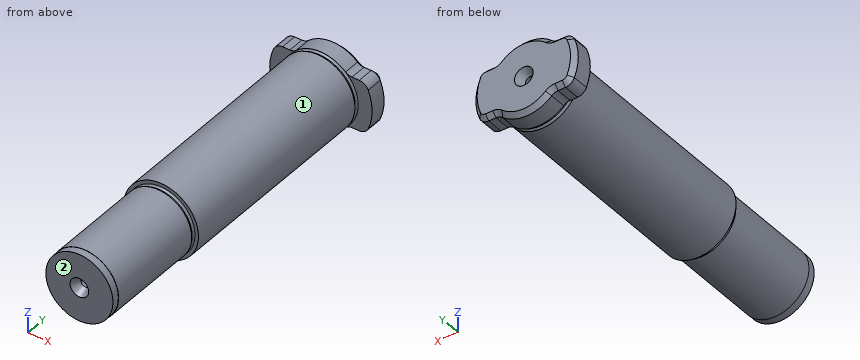
```python
from build123d import *

# Parameters (mm, degrees)
F0_R            = 11.4427
F1_DEPTH        = 2.54
F2_R            = 11.52271
F3_DEPTH        = 35.7378
F4_R            = 12.7
F4_R_2          = 11.52271
F5_DEPTH        = 74.7268
F7_DEPTH        = 7.1374
F8_T1_DEPTH     = 7.1374
F8_T3_DEPTH     = 18.5145836873
F9_SIZE         = 1.524
F13_D           = 3.048
F13_DEPTH       = 12.7
F13_CSINK_D     = 6.35
F13_CSINK_ANGLE = 60
F13_TIP         = 0.9157115834
F15_D           = 3.048
F15_DEPTH       = 12.7
F15_CSINK_D     = 6.35
F15_CSINK_ANGLE = 60
F15_TIP         = 0.9157115834


# Not quite as in the source:
# - a fillet or chamfer that OpenCascade refuses, or shapes differently, is made with other operations: its cross-section is extruded or revolved along the edge and cut away or added


with BuildPart() as f1:
    # F0 (on Front) → F1 (new body)
    with BuildSketch(Plane.XZ):
        Circle(F0_R)
    extrude(amount=-F1_DEPTH)

    # F2 (on face) → F3 (join)
    with BuildSketch(Plane(origin=(0, 2.54, 0), x_dir=(-1, 0, 0), z_dir=(0, 1, 0))):
        Circle(F2_R)
    extrude(amount=F3_DEPTH)

    # F4 (on face) → F5 (join)
    with BuildSketch(Plane(origin=(0, 38.2778, 0), x_dir=(-1, 0, 0), z_dir=(0, 1, 0))):
        Circle(F4_R)
        Circle(F4_R_2, mode=Mode.SUBTRACT)
        Circle(F4_R_2)
    extrude(amount=F5_DEPTH)

    # F6 (on face) → F7 (join)
    with BuildSketch(Plane(origin=(0, 113.0046, 0), x_dir=(-1, 0, 0), z_dir=(0, 1, 0))):
        with BuildLine():
            ThreePointArc((12.7, 0), (11.8067080769, 4.678850755), (9.2524969468, 8.6995))
            ThreePointArc((9.2524969468, 8.6995), (0, 12.7), (-9.2524969468, 8.6995))
            ThreePointArc((-9.2524969468, 8.6995), (-12.7, 0), (-9.2524969468, -8.6995))
            ThreePointArc((-9.2524969468, -8.6995), (0, -12.7), (9.2524969468, -8.6995))
            ThreePointArc((9.2524969468, -8.6995), (11.8067080769, -4.678850755), (12.7, 0))
        make_face()
        with BuildLine():
            ThreePointArc((15.126606354, -8.6995), (17.4498, 0), (15.126606354, 8.6995))
            Line((15.126606354, 8.6995), (9.2524969468, 8.6995))
            ThreePointArc((9.2524969468, 8.6995), (11.8067080769, 4.678850755), (12.7, 0))
            ThreePointArc((12.7, 0), (11.8067080769, -4.678850755), (9.2524969468, -8.6995))
            Line((9.2524969468, -8.6995), (15.126606354, -8.6995))
        make_face()
        with BuildLine():
            ThreePointArc((-9.2524969468, -8.6995), (-12.7, 0), (-9.2524969468, 8.6995))
            Line((-9.2524969468, 8.6995), (-15.126606354, 8.6995))
            ThreePointArc((-15.126606354, 8.6995), (-17.4498, 0), (-15.126606354, -8.6995))
            Line((-15.126606354, -8.6995), (-9.2524969468, -8.6995))
        make_face()
    extrude(amount=F7_DEPTH)

    # F8: fillet of radius 3.302 on 8 edges, made by hand

    # F8_s2 → F8_t1 (join)
    with BuildSketch(Plane.XZ.offset(-120.142)):
        with BuildLine():
            ThreePointArc((-8.4002604126, -9.525), (-9.4168948242, -8.9127618272), (-10.5843281199, -8.6995))
            Line((-10.5843281199, -8.6995), (-9.2524969468, -8.6995))
            ThreePointArc((-9.2524969468, -8.6995), (-8.8360241715, -9.1222078928), (-8.4002604126, -9.525))
        make_face()
        with BuildLine():
            ThreePointArc((8.4002604126, -9.525), (9.4168948242, -8.9127618272), (10.5843281199, -8.6995))
            Line((10.5843281199, -8.6995), (9.2524969468, -8.6995))
            ThreePointArc((9.2524969468, -8.6995), (8.8360241715, -9.1222078928), (8.4002604126, -9.525))
        make_face()
        with BuildLine():
            ThreePointArc((-8.4002604126, 9.525), (-9.4168948242, 8.9127618272), (-10.5843281199, 8.6995))
            Line((-10.5843281199, 8.6995), (-9.2524969468, 8.6995))
            ThreePointArc((-9.2524969468, 8.6995), (-8.8360241715, 9.1222078928), (-8.4002604126, 9.525))
        make_face()
        with BuildLine():
            ThreePointArc((8.4002604126, 9.525), (9.4168948242, 8.9127618272), (10.5843281199, 8.6995))
            Line((10.5843281199, 8.6995), (9.2524969468, 8.6995))
            ThreePointArc((9.2524969468, 8.6995), (8.8360241715, 9.1222078928), (8.4002604126, 9.525))
        make_face()
    extrude(amount=F8_T1_DEPTH)

    # F8_s4 → F8_t3 (cut)
    with BuildSketch(Plane.XZ.offset(-125.8305918437)):
        with BuildLine():
            ThreePointArc((-13.0777382827, -8.6995), (-14.913976773, -8.1418454969), (-16.1299931781, -6.6572396768))
            ThreePointArc((-16.1299931781, -6.6572396768), (-15.6616238106, -7.6947423385), (-15.126606354, -8.6995))
            Line((-15.126606354, -8.6995), (-13.0777382827, -8.6995))
        make_face()
        with BuildLine():
            ThreePointArc((13.0777382827, -8.6995), (14.913976773, -8.1418454969), (16.1299931781, -6.6572396768))
            ThreePointArc((16.1299931781, -6.6572396768), (15.6616238106, -7.6947423385), (15.126606354, -8.6995))
            Line((15.126606354, -8.6995), (13.0777382827, -8.6995))
        make_face()
        with BuildLine():
            ThreePointArc((-16.1299931781, 6.6572396768), (-14.913976773, 8.1418454969), (-13.0777382827, 8.6995))
            Line((-13.0777382827, 8.6995), (-15.126606354, 8.6995))
            ThreePointArc((-15.126606354, 8.6995), (-15.6616238106, 7.6947423385), (-16.1299931781, 6.6572396768))
        make_face()
        with BuildLine():
            ThreePointArc((16.1299931781, 6.6572396768), (14.913976773, 8.1418454969), (13.0777382827, 8.6995))
            Line((13.0777382827, 8.6995), (15.126606354, 8.6995))
            ThreePointArc((15.126606354, 8.6995), (15.6616238106, 7.6947423385), (16.1299931781, 6.6572396768))
        make_face()
    extrude(amount=F8_T3_DEPTH, mode=Mode.SUBTRACT)

    # F9
    f9_edges = [f1.edges().sort_by_distance(p)[0] for p in [
        (0, 120.142, 12.7),
        (0, 120.142, -12.7),
        (-9.416895, 120.142, -8.912762),
        (9.416895, 120.142, -8.912762),
        (11.831033, 120.142, -8.6995),
        (14.913977, 120.142, -8.141845),
        (17.4498, 120.142, 0),
        (14.913977, 120.142, 8.141845),
        (11.831033, 120.142, 8.6995),
        (9.416895, 120.142, 8.912762),
        (-9.416895, 120.142, 8.912762),
        (-11.831033, 120.142, 8.6995),
        (-14.913977, 120.142, 8.141845),
        (-17.4498, 120.142, 0),
        (-14.913977, 120.142, -8.141845),
        (-11.831033, 120.142, -8.6995),
    ]]
    chamfer(f9_edges, length=F9_SIZE)

    # F10 (on Top) → F11 (revolve, cut)
    with BuildSketch(Plane.XY):
        with BuildLine():
            Line((-12.7, 113.0046), (-12.7, 111.4806))
            Line((-12.7, 111.4806), (-12.2600590949, 112.2426))
            ThreePointArc((-12.2600590949, 112.2426), (-12.2600590949, 112.7506), (-12.7, 113.0046))
        make_face()
        with BuildLine():
            Line((11.52271, 36.7538), (11.52271, 38.2778))
            ThreePointArc((11.52271, 38.2778), (11.0827690949, 38.0238), (11.0827690949, 37.5158))
            Line((11.0827690949, 37.5158), (11.52271, 36.7538))
        make_face()
    revolve(axis=Axis((0, 32.0415347815, 0), (0, 1, 0)), mode=Mode.SUBTRACT)

    # F13
    with Locations(Plane.XZ):
        with Locations((0, 0)):
            CounterSinkHole(F13_D / 2, F13_CSINK_D / 2, depth=F13_DEPTH, counter_sink_angle=F13_CSINK_ANGLE)
            with Locations((0, 0, -(F13_DEPTH + F13_TIP / 2))):  # 118° drill point
                Cone(0, F13_D / 2, F13_TIP, mode=Mode.SUBTRACT)

    # F15
    with Locations(Plane(origin=(0, 120.142, 0), x_dir=(-1, 0, 0), z_dir=(0, 1, 0))):
        with Locations((0, 0)):
            CounterSinkHole(F15_D / 2, F15_CSINK_D / 2, depth=F15_DEPTH, counter_sink_angle=F15_CSINK_ANGLE)
            with Locations((0, 0, -(F15_DEPTH + F15_TIP / 2))):  # 118° drill point
                Cone(0, F15_D / 2, F15_TIP, mode=Mode.SUBTRACT)


solid = f1.part
```
The model under review builds one solid part; all positions refer to its coordinate system, in mm. Face numbers are marked on the shaded views. A direction names the side the tool comes from. Round coordinates to 2 decimals unless told otherwise and drop trailing zeros. Loops run counter-clockwise (first coordinate to the right, second up) from the corner with the lowest first, then second, coordinate; pieces in that order, holes last. Notation, with made-up numbers: M 40,67 L 98,67 A25 ccw 98,101 Z; hole C 53,49.5 d11. An arc over 180 degrees is marked long. Answer as a JSON object with one key per item and string values.
(1) To check wall thickness, follow line 1 along Z through (x, y) = (0, 114.25); line 2 along Z through (x, y) = (0, 10). State the ranges of each line that lie inside material, in increasing order.
Resolved:
{"line 1": "-12.7 to -1.52, 1.52 to 12.7", "line 2": "-11.52 to -1.52, 1.52 to 11.52"}
(2) Tool access review of the marked faces 1 and 2: name each direction out of +Z, -Z, +X, -X, +Y, -Y from which nothing blocks a thin tool from reaching the whole face with its end or side.
Resolved:
{"face 1": "-Y", "face 2": "+Z, -Z, +X, -X, -Y"}
(3) Take a section at B-B on y = 101. Give the boundary of the cut face in (x, z), and give its area (3 significant figures).
Resolved:
{"outline": "C 0,0 d25.4", "area": "507 mm²"}
(4) Clearance check with flat-ended pins moving along their axes: P1, Ø8, axis at y = 85.5, z = -5.5, coming from the +X side; P2, Ø1.2, axis at x = -12, y = 115, coming from the +Z side; P3, Ø10, axis at x = -13, z = -4.5, coming from the -Y side; P4, Ø8, axis at x = 12, y = 106, coming from the +Z side. State where each tip first meets the part, or that it passes through.
Resolved:
{"P1": "x = 12.61", "P2": "z = 8.7", "P3": "y = 0", "P4": "z = 9.86"}
(5) Take a section at A-A on y = 15. Give the boundary of the cut face in (x, z), and give its area (3 significant figures).
Resolved:
{"outline": "C 0,0 d23.05", "area": "417 mm²"}
